The listing builds one solid part. Answer for the finished solid, in the listing's coordinates (mm). Face numbers are marked on the shaded views. A direction names the side the tool comes from. Round coordinates to 2 decimals unless told otherwise and drop trailing zeros. Write each loop counter-clockwise with the first axis right and the second up, starting at its lowest first coordinate (ties: lowest second). Pieces come first, ordered by that corner, then holes. Notation, with made-up numbers: (79.25, 57.5) - (125.25, 57.5) arc R25 cw to (125.25, 78.5) - close; hole circle Ø11 at (58.25, -13.5). An arc over 180 degrees is marked (long way). Return JSON: item names as keys, results as strings. Group by question number.
(1) Each of these flat-tipped pins is pushed along its axis until it touches: pin 1 (3 mm diameter, centred on x = 37, z = 42, fed in from -Y); pin 2 (8 mm diameter, centred on x = 40, z = -27, fed in from -Y); pin 3 (6.5 mm diameter, centred on x = 23, z = 2, fed in from +Y). Where does it stop, or does it pass through?
(2) Section A-A, the plane x = 7.5 is taken. Write down the section's boundary in (y, z), then the cut area to 3 significant figures.
(3) Which of the six approach directions +Z, -Z, +X, -X, +Y, -Y give full straight-line access (tool end or side, diameter ignored) to the marked faces 1, 2 and 3?
(4) Find the intervals of material crossed by line 1 along X through (y, z) = (40, -10); line 2 along X through (y, z) = (18, 42.5); line 3 along Z through (x, y) = (26.5, -1), in increasing order. Write a range as [from, to].
(5) Determine the mould class of the marked faces 4, 5 and 6 for opening direction Z: +Z half, -Z half, draft (parallel to the pull), parting line (faces both ways), or undercut.
(6) Section D-D, the plane x = 42 is taken. Write down the section's boundary in (y, z), then the cut area to 3 significant figures.
```python
from build123d import *

# Parameters (mm, degrees)
CHAMFER_1_SIZE      = 1
SKETCH_3_W          = 20
SKETCH_3_H          = 8.011692653
SKETCH_4_W          = 8
SKETCH_4_H          = 6.987786138
CUT_EXTRUDE_1_DEPTH = 96.45941546


with BuildPart() as part:
    # 草图1 → 旋转1 (revolve)
    with BuildSketch(Plane.XY, mode=Mode.PRIVATE) as revolve_1_sk:
        Polygon((0, 27.5), (0, 57.5), (12, 57.5), (12, 52.5), (6, 52.5), (6, 43), (12, 43), (12, 40), (50, 40), (50, 27.5), align=None)
    revolve(revolve_1_sk.sketch.rotate(Axis((0, 0, 0), (1, 0, 0)), 90), axis=Axis((0, 0, 0), (1, 0, 0)))

    # 倒角1
    chamfer_1_edges = [part.edges().sort_by_distance(p)[0] for p in [
        (0, 0, -27.5),
        (50, 0, -27.5),
    ]]
    chamfer(chamfer_1_edges, length=CHAMFER_1_SIZE)

    # 草图3 → 旋转2 (revolve)
    with BuildSketch(Plane.XY, mode=Mode.PRIVATE) as revolve_2_sk:
        with Locations((37, 43.994153674)):
            Rectangle(SKETCH_3_W, SKETCH_3_H)
    revolve(revolve_2_sk.sketch.rotate(Axis((27, 0, 0), (1, 0, 0)), 90), axis=Axis((27, 0, 0), (1, 0, 0)))

    # 草图4 → 切除-拉伸1 (cut, through all)
    with BuildSketch(Plane.ZY):
        with Locations((0, -25.606106931)):
            Rectangle(SKETCH_4_W, SKETCH_4_H)
    extrude(amount=-CUT_EXTRUDE_1_DEPTH, mode=Mode.SUBTRACT)


solid = part.part
```
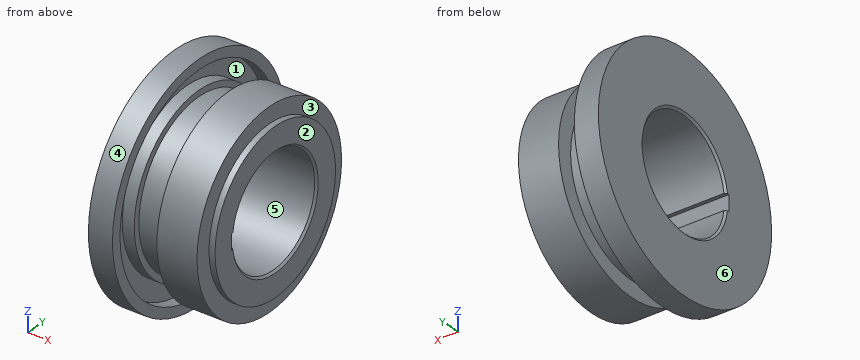
Working result:
{
 "1": {"pin 1": "stops at y = -25.76", "pin 2": "stops at y = -42.13", "pin 3": "stops at y = 40"},
 "2": {"outline": "circle Ø115 at (0, 0); circle Ø86 at (0, 0); hole circle Ø105 at (0, 0); hole (-29.1, -4) - (-27.21, -4) arc R27.5 ccw (long way) to (-27.21, 4) - (-29.1, 4) - close", "area": "5,150 mm^2"},
 "3": {"face 1": "none", "face 2": "+Z, -Z, +X, +Y, -Y", "face 3": "+X"},
 "4": {"line 1": "x = [0, 12], [27, 47]", "line 2": "x = [0, 6], [27, 47]", "line 3": "z = [-39.99, -27.48], [27.48, 39.99]"},
 "5": {"face 4": "parting line", "face 5": "undercut", "face 6": "draft"},
 "6": {"outline": "circle Ø96 at (0, 0); hole (-29.1, -4) - (-27.21, -4) arc R27.5 ccw (long way) to (-27.21, 4) - (-29.1, 4) - close", "area": "4,850 mm^2"}
}
